from build123d import *

# Parameters (mm, degrees)
F0_W         = 40.64
F0_H         = 40.64
F1_DEPTH     = 44.45
F2_T         = -1.27
F3_T1_DEPTH  = 38.1
F3_T3_DEPTH  = 38.1
F3_T9_DEPTH  = 51.1641495789
F3_T15_DEPTH = 51.1641495789
F3_T24_DEPTH = 51.1641495789
F3_T30_DEPTH = 51.1641495789
F3_T39_DEPTH = 51.1641495789
F3_T45_DEPTH = 51.1641495789
F3_T54_DEPTH = 51.1641495789
F3_T60_DEPTH = 51.1641495789


# Not quite as in the source:
# - a fillet or chamfer that OpenCascade refuses, or shapes differently, is made with other operations: its cross-section is extruded or revolved along the edge and cut away or added


with BuildPart() as f1:
    # F0 (on Top) → F1 (new body)
    with BuildSketch(Plane.XY):
        with Locations((-1.2905509211, 8.1801498235)):
            Rectangle(F0_W, F0_H)
    extrude(amount=F1_DEPTH)

    # F2
    f2_openings = [f1.faces().sort_by_distance(p)[0] for p in [
        (-1.290551, 8.18015, 44.45),
    ]]
    offset(amount=F2_T, openings=f2_openings)

    # F3: chamfer of 5.08 on 4 edges, made by hand

    # F3_s2 → F3_t1 (cut)
    with BuildSketch(Plane.XZ.offset(-27.2301498235)):
        Polygon((-25.4205509211, 44.45), (-20.3405509211, 39.37), (-20.3405509211, 44.45), align=None)
        Polygon((22.8394490789, 44.45), (17.7594490789, 39.37), (17.7594490789, 44.45), align=None)
    extrude(amount=F3_T1_DEPTH, mode=Mode.SUBTRACT)

    # F3_s4 → F3_t3 (cut)
    with BuildSketch(Plane.YZ.offset(-20.3405509211)):
        Polygon((32.3101498235, 44.45), (27.2301498235, 39.37), (27.2301498235, 44.45), align=None)
        Polygon((-15.9498501765, 44.45), (-10.8698501765, 39.37), (-10.8698501765, 44.45), align=None)
    extrude(amount=F3_T3_DEPTH, mode=Mode.SUBTRACT)


with BuildPart() as f3_tool7:
    # F3_s8 → F3_t9 (new body)
    with BuildSketch(Plane.YZ.offset(17.7594490789)):
        Polygon((32.3101498235, 44.45), (27.2301498235, 39.37), (27.2301498235, 44.45), align=None)
    extrude(amount=-F3_T9_DEPTH)

    split(bisect_by=Plane.XZ.offset(-28.5001498235), keep=Keep.TOP)

    split(bisect_by=Plane.YZ.offset(-21.6105509211), keep=Keep.TOP)

    split(bisect_by=Plane.YZ.offset(-20.3405509211), keep=Keep.BOTTOM)


with BuildPart() as f3_tool13:
    # F3_s14 → F3_t15 (new body)
    with BuildSketch(Plane.XZ.offset(-40.2942994024)):
        Polygon((-25.4205509211, 44.45), (-20.3405509211, 39.37), (-20.3405509211, 44.45), align=None)
    extrude(amount=F3_T15_DEPTH)

    split(bisect_by=Plane.XZ.offset(-28.5001498235), keep=Keep.TOP)

    split(bisect_by=Plane.YZ.offset(-21.6105509211), keep=Keep.TOP)

    split(bisect_by=Plane.XZ.offset(-27.2301498235), keep=Keep.BOTTOM)


with BuildPart() as f3_tool7_1:
    add(f3_tool7.part)

    # F3_t19: intersect F3_tool13
    add(f3_tool13.part, mode=Mode.INTERSECT)


with BuildPart() as f1_1:
    add(f1.part)

    # F3_t5: cut F3_tool7
    add(f3_tool7_1.part, mode=Mode.SUBTRACT)


with BuildPart() as f3_tool22:
    # F3_s23 → F3_t24 (new body)
    with BuildSketch(Plane.YZ.offset(-33.4047005)):
        Polygon((-15.9498501765, 44.45), (-10.8698501765, 39.37), (-10.8698501765, 44.45), align=None)
    extrude(amount=F3_T24_DEPTH)

    split(bisect_by=Plane.YZ.offset(-21.6105509211), keep=Keep.TOP)

    split(bisect_by=Plane.XZ.offset(12.1398501765), keep=Keep.BOTTOM)

    split(bisect_by=Plane.YZ.offset(-20.3405509211), keep=Keep.BOTTOM)


with BuildPart() as f3_tool28:
    # F3_s29 → F3_t30 (new body)
    with BuildSketch(Plane.XZ.offset(-27.2301498235)):
        Polygon((-25.4205509211, 44.45), (-20.3405509211, 39.37), (-20.3405509211, 44.45), align=None)
    extrude(amount=F3_T30_DEPTH)

    split(bisect_by=Plane.YZ.offset(-21.6105509211), keep=Keep.TOP)

    split(bisect_by=Plane.XZ.offset(12.1398501765), keep=Keep.BOTTOM)

    split(bisect_by=Plane.XZ.offset(10.8698501765), keep=Keep.TOP)


with BuildPart() as f3_tool22_1:
    add(f3_tool22.part)

    # F3_t34: intersect F3_tool28
    add(f3_tool28.part, mode=Mode.INTERSECT)


with BuildPart() as f1_2:
    add(f1_1.part)

    # F3_t20: cut F3_tool22
    add(f3_tool22_1.part, mode=Mode.SUBTRACT)


with BuildPart() as f3_tool37:
    # F3_s38 → F3_t39 (new body)
    with BuildSketch(Plane.YZ.offset(30.8235986578)):
        Polygon((32.3101498235, 44.45), (27.2301498235, 39.37), (27.2301498235, 44.45), align=None)
    extrude(amount=-F3_T39_DEPTH)

    split(bisect_by=Plane.XZ.offset(-28.5001498235), keep=Keep.TOP)

    split(bisect_by=Plane.YZ.offset(19.0294490789), keep=Keep.BOTTOM)

    split(bisect_by=Plane.YZ.offset(17.7594490789), keep=Keep.TOP)


with BuildPart() as f3_tool43:
    # F3_s44 → F3_t45 (new body)
    with BuildSketch(Plane.XZ.offset(10.8698501765)):
        Polygon((22.8394490789, 44.45), (17.7594490789, 39.37), (17.7594490789, 44.45), align=None)
    extrude(amount=-F3_T45_DEPTH)

    split(bisect_by=Plane.XZ.offset(-28.5001498235), keep=Keep.TOP)

    split(bisect_by=Plane.YZ.offset(19.0294490789), keep=Keep.BOTTOM)

    split(bisect_by=Plane.XZ.offset(-27.2301498235), keep=Keep.BOTTOM)


with BuildPart() as f3_tool37_1:
    add(f3_tool37.part)

    # F3_t49: intersect F3_tool43
    add(f3_tool43.part, mode=Mode.INTERSECT)


with BuildPart() as f1_3:
    add(f1_2.part)

    # F3_t35: cut F3_tool37
    add(f3_tool37_1.part, mode=Mode.SUBTRACT)


with BuildPart() as f3_tool52:
    # F3_s53 → F3_t54 (new body)
    with BuildSketch(Plane.XZ.offset(23.9339997554)):
        Polygon((22.8394490789, 44.45), (17.7594490789, 39.37), (17.7594490789, 44.45), align=None)
    extrude(amount=-F3_T54_DEPTH)

    split(bisect_by=Plane.XZ.offset(12.1398501765), keep=Keep.BOTTOM)

    split(bisect_by=Plane.YZ.offset(19.0294490789), keep=Keep.BOTTOM)

    split(bisect_by=Plane.XZ.offset(10.8698501765), keep=Keep.TOP)


with BuildPart() as f3_tool58:
    # F3_s59 → F3_t60 (new body)
    with BuildSketch(Plane.YZ.offset(-20.3405509211)):
        Polygon((-15.9498501765, 44.45), (-10.8698501765, 39.37), (-10.8698501765, 44.45), align=None)
    extrude(amount=F3_T60_DEPTH)

    split(bisect_by=Plane.XZ.offset(12.1398501765), keep=Keep.BOTTOM)

    split(bisect_by=Plane.YZ.offset(19.0294490789), keep=Keep.BOTTOM)

    split(bisect_by=Plane.YZ.offset(17.7594490789), keep=Keep.TOP)


with BuildPart() as f3_tool52_1:
    add(f3_tool52.part)

    # F3_t64: intersect F3_tool58
    add(f3_tool58.part, mode=Mode.INTERSECT)


with BuildPart() as f1_4:
    add(f1_3.part)

    # F3_t50: cut F3_tool52
    add(f3_tool52_1.part, mode=Mode.SUBTRACT)


solid = f1_4.part
Verification items for the finished model (mm, model axes). A direction names the side the tool comes from. Give positions to 0.01 mm unless a question says otherwise; leave off trailing zeros. Loops run counter-clockwise (first coordinate to the right, second up) from the corner with the lowest first, then second, coordinate; pieces in that order, holes last. Notation, with made-up numbers: (38, -14) - (77, -14) arc R11 cw to (77, -9) - close; hole circle Ø4 at (15, 65). An arc over 180 degrees is marked (long way). Write each question's results on one line, items separated by ' | '.
1) Depth check by flat-ended pin: P1, Ø19, axis at x = -9, y = 9, coming from the +Z side; P2, Ø12, axis at x = 1, y = -1.5, coming from the -Z side. Enter the tip coordinate at first touch or a pass-through.
Solution:
P1: z = 1.27 | P2: z = 0
2) Sectioned sample at B-B on z = 6. Record the boundary of the cut face in (x, y).
Solution:
outline: (-21.61, -12.14) - (19.03, -12.14) - (19.03, 28.5) - (-21.61, 28.5) - close; hole (-20.34, -10.87) - (17.76, -10.87) - (17.76, 27.23) - (-20.34, 27.23) - close
3) Mould release check, pull along Y, two halves, no side actions. Record for faces 1 (the flat face through (18.4, 7.9, 40.01)), 2 (the flat face through (-2, 8, 0)), 3 (the flat face through (-2, 28.5, 20)): pulls with the +Y half, pulls with the -Y half, needs draft (parallel to the pull), parting line crosses it, or undercut.
Solution:
face 1: undercut | face 2: needs draft | face 3: pulls with the +Y half
4) Tool access check on faces 4 (the flat face through (19.029, 8, 20)), 5 (the flat face through (-20.98, 8.46, 40.01)). Record the directions out of +Z, -Z, +X, -X, +Y, -Y that give a thin tool (end or side, any length) a straight path to the whole face; none if there is none.
Solution:
face 4: +Z, -Z, +X, +Y, -Y | face 5: +Z
5) Sectioned sample at A-A on x = -6. Record the boundary of the cut face in (y, z), plus the area to 3 significant figures.
Solution:
outline: (-12.14, 0) - (28.5, 0) - (28.5, 40.64) - (27.23, 39.37) - (27.23, 1.27) - (-10.87, 1.27) - (-10.87, 39.37) - (-12.14, 40.64) - close | area: 150 mm2
6) Sectioned sample at C-C on y = 24. Record the boundary of the cut face in (x, z), plus the area to 3 significant figures.
Solution:
outline: (-21.61, 0) - (19.03, 0) - (19.03, 40.64) - (17.76, 39.37) - (17.76, 1.27) - (-20.34, 1.27) - (-20.34, 39.37) - (-21.61, 40.64) - close | area: 150 mm2
7) Material ranges on L1, parallel to X at y = 8.5, z = 24; L2, parallel to Y at x = -3, z = 37.5; L3, parallel to Z at x = 10, y = 5.5, recorded low to high. Write a range as from..to.
Solution:
L1: -21.61..-20.34, 17.76..19.03 | L2: -12.14..-10.87, 27.23..28.5 | L3: 0..1.27
